Could you check a few things on this drawing? It's one solid part, dimensions in mm from its lowest x, y, z. Coordinates: 2 decimals unless noted, no trailing zeros. Write each loop counter-clockwise with the first axis right and the second up, starting at its lowest first coordinate (ties: lowest second). Pieces come first, ordered by that corner, then holes.
Item 1: Please list where these lines run through material, in increasing order: line 1 (X direction, y = 22.5, z = 0.7); line 2 (Y direction, x = 23, z = 0.25); line 3 (X direction, y = 8.5, z = 0.25).
Item 2: I want a section at A-A (z = 0.5). Please give me the cut outline in (x, y) (3 decimals).
Item 3: I'm going to push flat-ended pins straight in: P1, Ø2.5, axis at x = 22.535, y = 22.535, coming from the -Z side; P2, Ø4.5, axis at x = 22.535, y = 7.465, coming from the +Z side. Where does each tip first touch, or does it pass through?
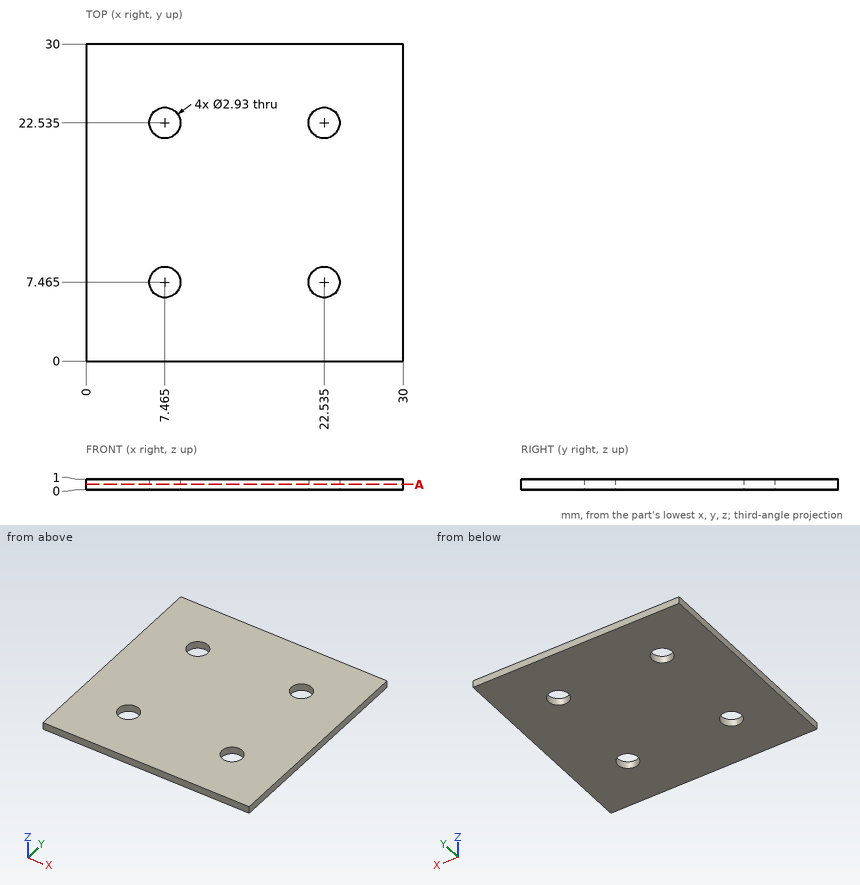
Answer:
1. line 1: x = 0 to 6, 8.93 to 21.07, 24 to 30
1. line 2: y = 0 to 6.08, 8.85 to 21.15, 23.92 to 30
1. line 3: x = 0 to 6.43, 8.5 to 21.5, 23.57 to 30
2. outline: (0, 0) - (30, 0) - (30, 30) - (0, 30) - close; hole circle Ø2.93 at (7.465, 7.465); hole circle Ø2.93 at (7.465, 22.535); hole circle Ø2.93 at (22.535, 7.465); hole circle Ø2.93 at (22.535, 22.535)
3. P1: passes through
3. P2: stops at z = 1
